from build123d import *

# Parameters (mm, degrees)
SKETCH1_W               = 13.1
SKETCH1_H               = 5.8
BOSS_EXTRUDE1_DEPTH     = 5
SKETCH10_W              = 5.65
SKETCH10_H              = 4.6
CUT_EXTRUDE7_DEPTH      = 6.6
SKETCH9_R               = 0.75
CUT_EXTRUDE6_DEPTH      = 6
CUT_EXTRUDE6_DEPTH_BACK = 6
BOSS_EXTRUDE2_START     = -5
BOSS_EXTRUDE2_DEPTH     = 10
SKETCH12_W              = 5.65
SKETCH12_H              = 4.6
SKETCH12_R              = 0.75
BOSS_EXTRUDE3_DEPTH     = 3.4


with BuildPart() as part:
    # Sketch1 → Boss-Extrude1 (new body, symmetric)
    with BuildSketch(Plane(origin=(0, 0, 0), x_dir=(1, 0, 0), z_dir=(0, 1, 0))):
        Rectangle(SKETCH1_W, SKETCH1_H)
    extrude(amount=BOSS_EXTRUDE1_DEPTH, both=True)

    # Sketch10 → Cut-Extrude7 (cut)
    with BuildSketch(Plane(origin=(0, 5, 0), x_dir=(1, 0, 0), z_dir=(0, 1, 0))):
        with Locations((-3.125, 0)):
            Rectangle(SKETCH10_W, SKETCH10_H)
        with Locations((3.125, 0)):
            Rectangle(SKETCH10_W, SKETCH10_H)
    extrude(amount=-CUT_EXTRUDE7_DEPTH, mode=Mode.SUBTRACT)

    # Sketch9 → Cut-Extrude6 (cut, two sides)
    with BuildSketch(Plane(origin=(0, 0, 0), x_dir=(1, 0, 0), z_dir=(0, 1, 0))) as cut_extrude6_sk:
        with Locations((-4.625, 0)):
            Circle(SKETCH9_R)
        with Locations((-1.625, 0)):
            Circle(SKETCH9_R)
        with Locations((1.625, 0)):
            Circle(SKETCH9_R)
        with Locations((4.625, 0)):
            Circle(SKETCH9_R)
    extrude(amount=CUT_EXTRUDE6_DEPTH, mode=Mode.SUBTRACT)
    extrude(cut_extrude6_sk.sketch, amount=-CUT_EXTRUDE6_DEPTH_BACK, mode=Mode.SUBTRACT)

    # Sketch11 → Boss-Extrude2 (add)
    with BuildSketch(Plane(origin=(0, 0, 0), x_dir=(1, 0, 0), z_dir=(0, 1, 0)).offset(BOSS_EXTRUDE2_START)):
        Polygon((-3.425, 8.1), (-3.425, 2.9), (-2.825, 2.9), (-2.825, 7.5), (2.825, 7.5), (2.825, 2.9), (3.425, 2.9), (3.425, 8.1), align=None)
    extrude(amount=BOSS_EXTRUDE2_DEPTH)

    # Sketch12 → Boss-Extrude3 (add)
    with BuildSketch(Plane.XZ.offset(5)):
        with Locations((0, -5.2)):
            Rectangle(SKETCH12_W, SKETCH12_H)
        with Locations((-1.5, -5.2)):
            Circle(SKETCH12_R, mode=Mode.SUBTRACT)
        with Locations((1.5, -5.2)):
            Circle(SKETCH12_R, mode=Mode.SUBTRACT)
    extrude(amount=-BOSS_EXTRUDE3_DEPTH)


solid = part.part
Read the model definition and answer for the solid it produces. Units are mm, in the model's axes. A direction names the side the tool comes from. Round coordinates to 2 decimals unless told otherwise and drop trailing zeros. Loops run counter-clockwise (first coordinate to the right, second up) from the corner with the lowest first, then second, coordinate; pieces in that order, holes last. Notation, with made-up numbers: (54.25, -1) - (75.25, -1) arc R18 cw to (75.25, 5) - close; hole circle Ø4 at (88.25, 89). An arc over 180 degrees is marked (long way). One line per question, with ' | ' between items. Start each with the question number.
Q1. Section B-B on y = -2 is taken. Give the vertices of the cut face in (x, z) (3 decimals), plus the area to 3 significant figures.
Q2. Find the intervals of material crossed by L1, parallel to X at y = -1.5, z = 1.5; L2, parallel to Z at x = 1.5, y = -0.5; L3, parallel to X at y = -3.7, z = 0 (3 decimals), in increasing order.
Q3. For a pull along X with two mould halves and no side action, classify faces 4 (the flat face through (3.425, 0, -5)), 5 (the flat face through (0, 0, 2.9)), 6 (the flat face through (2.825, 2, -5)) as +X half, -X half, draft (parallel to the pull), parting line (faces both ways), or undercut.
Q4. Section D-D on y = 4 is taken. Give the vertices of the cut face in (x, z) (3 decimals), plus the area to 3 significant figures.
Q5. Section C-C on z = -5.2 is taken. Give the vertices of the cut face in (x, y) (3 decimals), plus the area to 3 significant figures.
Q6. For faces 1 (the flat face through (-3.425, 0, -6)), 2 (the flat face through (0.3, 2, 0)), 3 (the flat face through (0, 0, -8.1)), determine the directions among +Z, -Z, +X, -X, +Y, -Y from which every point of the face is accessible in a straight line to the end or side of a thin tool.
Q7. Section A-A on z = 0 is taken. Give the vertices of the cut face in (x, y) (3 decimals).
Q8. Flat-ended cylindrical pins translate along their axes: pin 1 (1.6 mm diameter, centred on x = 6, y = 0.5, fed in from -Z); pin 2 (1 mm diameter, centred on y = -3.5, z = -4.5, fed in from -X) (3 decimals); pin 3 (1.7 mm diameter, centred on x = 1.625, z = 0, fed in from +Y). Find the tip coordinate at first contact, or state that the pin passes through.
Established:
1) outline: (-6.55, -2.9) - (-3.425, -2.9) - (-3.425, -8.1) - (3.425, -8.1) - (3.425, -2.9) - (6.55, -2.9) - (6.55, 2.9) - (-6.55, 2.9) - close; hole circle Ø1.5 at (-4.625, 0); hole circle Ø1.5 at (-1.625, 0); hole circle Ø1.5 at (-1.5, -5.2); hole circle Ø1.5 at (1.5, -5.2); hole circle Ø1.5 at (1.625, 0); hole circle Ø1.5 at (4.625, 0) | area: 101 mm²
2) L1: -6.55 to -5.95, -0.3 to 0.3, 5.95 to 6.55 | L2: -8.1 to -7.5, -2.9 to -2.3, 2.3 to 2.9 | L3: -6.55 to -5.375, -3.875 to -2.375, -0.875 to 0.875, 2.375 to 3.875, 5.375 to 6.55
3) face 4: +X half | face 5: draft | face 6: undercut
4) outline: (-6.55, -2.9) - (-3.425, -2.9) - (-3.425, -8.1) - (3.425, -8.1) - (3.425, -2.9) - (6.55, -2.9) - (6.55, 2.9) - (-6.55, 2.9) - close; hole (-5.95, -2.3) - (-0.3, -2.3) - (-0.3, 2.3) - (-5.95, 2.3) - close; hole (-2.825, -7.5) - (2.825, -7.5) - (2.825, -2.9) - (-2.825, -2.9) - close; hole (0.3, -2.3) - (5.95, -2.3) - (5.95, 2.3) - (0.3, 2.3) - close | area: 33.6 mm²
5) outline: (-3.425, -5) - (-2.25, -5) - (-2.25, -1.6) - (-2.825, -1.6) - (-2.825, 5) - (-3.425, 5) - close; (-0.75, -5) - (0.75, -5) - (0.75, -1.6) - (-0.75, -1.6) - close; (2.25, -5) - (3.425, -5) - (3.425, 5) - (2.825, 5) - (2.825, -1.6) - (2.25, -1.6) - close | area: 21.0 mm²
6) face 1: -Z, -X, +Y, -Y | face 2: +Y | face 3: -Z, +X, -X, +Y, -Y
7) outline: (-6.55, -5) - (-5.375, -5) - (-5.375, -1.6) - (-5.95, -1.6) - (-5.95, 5) - (-6.55, 5) - close; (-3.875, -5) - (-2.375, -5) - (-2.375, -1.6) - (-3.875, -1.6) - close; (-0.875, -5) - (0.875, -5) - (0.875, -1.6) - (0.3, -1.6) - (0.3, 5) - (-0.3, 5) - (-0.3, -1.6) - (-0.875, -1.6) - close; (2.375, -5) - (3.875, -5) - (3.875, -1.6) - (2.375, -1.6) - close; (5.375, -5) - (6.55, -5) - (6.55, 5) - (5.95, 5) - (5.95, -1.6) - (5.375, -1.6) - close
8) pin 1: z = -2.9 | pin 2: x = -3.425 | pin 3: y = -1.6
